```python
from build123d import *

# Parameters (mm, degrees)
F0_R     = 2.4977360004
F1_DEPTH = 60


with BuildPart() as f1:
    # F0 (on Top) → F1 (new body, symmetric)
    with BuildSketch(Plane.XY):
        Circle(F0_R)
    extrude(amount=F1_DEPTH, both=True)

    # F2 (on Front) → F3 (revolve)
    with BuildSketch(Plane.XZ):
        with BuildLine():
            Line((0, 0), (0, 63.1117001176))
            add(Edge.make_bspline(
                [(0, 63.1117001176), (-8.564592389, 59.3954542786), (-28.7472157674, 50.6380509202), (-22.5542900222, 18.5000735529), (-18.9893618226, 0)],
                knots=[0, 0, 0, 0, 0.4243547644, 1, 1, 1, 1], degree=3))
            Line((-18.9893618226, 0), (0, 0))
        make_face()
    revolve(axis=Axis((0, 0, 31.5558500588), (0, 0, 1)))

    # F4 (on Front) → F5 (revolve)
    with BuildSketch(Plane.XZ):
        Polygon((9.49467998, 0), (0, 0), (0, -19.547874108), (39.3750034273, -19.547874108), (39.3750034273, -16.1968097091), (26.8085133284, -16.1968097091), (26.8085133284, -13.1250005215), (17.3138324171, -13.1250005215), (17.3138324171, -6.9813835435), (9.49467998, -6.9813835435), align=None)
    revolve(axis=Axis((0, 0, -9.773937054), (0, 0, 1)))


solid = f1.part
```
Work out the finished part from the listing and answer in its coordinate system (mm). A direction names the side the tool comes from. Round coordinates to 2 decimals unless told otherwise and drop trailing zeros. Order: outer loops, then holes, each group sorted by start corner. A loop starts at its lowest first (then second) coordinate and runs counter-clockwise, first axis right, second up.
Q1. A cutting plane is placed at A-A, the plane y = 34.5. Determine the outline of the cut face in (x, z).
Solution:
outline: (-18.98, -19.55) - (18.98, -19.55) - (18.98, -16.2) - (-18.98, -16.2) - close
Q2. A tool of negligible diameter and unlimited length cuts with its end or side. For faces 4 (the cylindrical face through (1.34, 2.11, -39.49)), 5 (the cylindrical face through (14.412, 22.605, -14.639)), 6 (the cylindrical face through (-6.998, 6.417, -3.442)), from which of +Z, -Z, +X, -X, +Y, -Y can it reach the whole face along a straight path? Write none if from no direction.
Solution:
face 4: -Z
face 5: +Z
face 6: none
Q3. Given pin 1 Ø4 at (x, y) = (-8.5, 12.5) entering from +Z; pin 2 Ø12 at (x, y) = (1.5, 31.5) entering from -Z; pin 3 Ø12 at (x, y) = (-19.5, 2) entering from +Z, each flat-ended and moving along its own axis, determine where each tip first touches the part or whether it passes through.
Solution:
pin 1: stops at z = 56.44
pin 2: stops at z = -19.55
pin 3: stops at z = 56.09
Q4. The mould has two halves that part along Z. Classify faces 1 (the flat face through (-0.4, -17.5, -13.125)), 2 (the flat face through (-8, 1, -19.548)), 3 (the flat face through (8, -26, -16.197)): pulls with the +Z half, pulls with the -Z half, needs draft (parallel to the pull), parting line crosses it, or undercut.
Solution:
face 1: undercut
face 2: pulls with the -Z half
face 3: pulls with the +Z half
Q5. A cutting plane is placed at B-B, the plane z = -24. Determine the outline of the cut face in (x, y).
Solution:
outline: circle Ø5 at (0, 0)
Q6. Find the intervals of material crossed by line 1 along Z through (x, y) = (17, 4) (3 decimals); line 2 along Z through (x, y) = (-23.5, 9.5) (3 decimals); line 3 along Z through (x, y) = (20, 20), in increasing order.
Solution:
line 1: z = -19.548 to -13.125, 0 to 52.767
line 2: z = -19.548 to -13.125
line 3: z = -19.55 to -16.2
